The listing builds one solid part. Answer for the finished solid, in the listing's coordinates (mm). A direction names the side the tool comes from. Give positions to 0.01 mm unless a question says otherwise; leave off trailing zeros. Order: outer loops, then holes, each group sorted by start corner. A loop starts at its lowest first (then second) coordinate and runs counter-clockwise, first axis right, second up. Notation, with made-up numbers: (-31.5, 57) - (-15.5, 57) arc R34 ccw to (-15.5, 94) - close; hole circle Ø11 at (28, -0.5). An arc over 180 degrees is marked (long way). Answer as CSV lines item,"result". Start each with the question number.
1. Flat-ended cylindrical pins translate along their axes: pin 1 (0.5 mm diameter, centred on x = -3.5, y = -2, fed in from +Z); pin 2 (1.5 mm diameter, centred on x = -13, y = -2.5, fed in from -Z); pin 3 (2 mm diameter, centred on x = 32.5, y = -2, fed in from -Z); pin 4 (8 mm diameter, centred on x = -16, z = -41.5, fed in from -Y). Find the tip coordinate at first contact, or state that the pin passes through.
2. Which of the six approach directions +Z, -Z, +X, -X, +Y, -Y give full straight-line access (tool end or side, diameter ignored) to faces 1 (the cylindrical face through (-31.83, -3.05, 35.2)), 2 (the cylindrical face through (38.398, -0.673, -21.926)), 3 (the flat face through (0, -2, 46.1)), 4 (the cylindrical face through (31.83, -3.05, -35.2)), 5 (the flat face through (37.994, -0.159, -21.693))?
3. Section B-B on y = 1 is taken. Give the vertices of the cut face in (x, z) (3 decimals).
4. Determine the mould class of faces 6 (the flat face through (-39, -3.5, -23)), 7 (the flat face through (-38.347, -1.743, -22.382)), 8 (the conical face through (-22.56, 0.57, -38.24)) for opening direction Y: +Y half, -Y half, draft (parallel to the pull), parting line (faces both ways), or undercut.
5. Section A-A on x = 0 is taken. Give the vertices of the cut face in (y, z).
6. Section C-C on z = 0 is taken. Give the vertices of the cut face in (x, y).
7. Consider line 1 along Z through (x, y) = (7.5, -1.5); line 2 along X through (y, z) = (0.9, 0); line 3 along X through (y, z) = (0.7, 0). Determine where each line is inside the solid, lowest interval first. Write a range as [from, to].
from build123d import *

# Parameters (mm, degrees)
BOSS_EXTRUDE2_START       = -3.5
SKETCH1_W                 = 30
SKETCH1_H                 = 2.35
BOSS_EXTRUDE2_DEPTH       = 4.5
SKETCH3_R                 = 52.5
SKETCH3_R_2               = 42
SKETCH3_R_3               = 1.5
BOSS_EXTRUDE3_DEPTH       = 2
CHAMFER1_SIZE             = 3
CHAMFER1_SIZE_2           = 0.803847577
FILLET1_R                 = 1.5
F_1_0MM_START             = -15
F_1_0MM_DOWEL_SLOT1_DEPTH = 30
CIRPATTERN1_COUNT         = 6
FILLET1_OF_CIRPATTERN1_R  = 1.5


# Read off the part's stored shape, not the designer's step: Ø1.0mm Dowel Slot1
with BuildPart() as part:
    # Sketch1 → Boss-Extrude2 (new body)
    with BuildSketch(Plane(origin=(0, 0, 0), x_dir=(1, 0, 0), z_dir=(0, 1, 0)).offset(BOSS_EXTRUDE2_START)):
        with Locations((0, -44.925)):
            Rectangle(SKETCH1_W, SKETCH1_H)
    boss_extrude2 = extrude(amount=BOSS_EXTRUDE2_DEPTH)

    # Sketch3 → Boss-Extrude3 (add)
    with BuildSketch(Plane(origin=(0, 0, 0), x_dir=(1, 0, 0), z_dir=(0, 1, 0))):
        with Locations(Location((0, 0, 0), (0, 0, 270))):
            Circle(SKETCH3_R)
        with Locations(Location((0, 0, 0), (0, 0, 270))):
            Circle(SKETCH3_R_2, mode=Mode.SUBTRACT)
        with Locations(Location((-23.135, 40.070995433, 0), (0, 0, 270))):
            Circle(SKETCH3_R_3, mode=Mode.SUBTRACT)
        with Locations(Location((23.135, 40.070995433, 0), (0, 0, 270))):
            Circle(SKETCH3_R_3, mode=Mode.SUBTRACT)
        with Locations(Location((46.27, 0, 0), (0, 0, 270))):
            Circle(SKETCH3_R_3, mode=Mode.SUBTRACT)
        with Locations(Location((23.135, -40.070995433, 0), (0, 0, 270))):
            Circle(SKETCH3_R_3, mode=Mode.SUBTRACT)
        with Locations(Location((-23.135, -40.070995433, 0), (0, 0, 270))):
            Circle(SKETCH3_R_3, mode=Mode.SUBTRACT)
        with Locations(Location((-46.27, 0, 0), (0, 0, 270))):
            Circle(SKETCH3_R_3, mode=Mode.SUBTRACT)
    extrude(amount=BOSS_EXTRUDE3_DEPTH)

    # Chamfer1
    # the kernel refuses this chamfer: 3, 0.803847577 mm, written as the material it takes off along each edge
    with BuildSketch(Plane(origin=(23.135, 2, 40.070995433), x_dir=(0, 0, 1), z_dir=(-1, 0, 0))) as chamfer1_piece_1:
        Polygon((1.5, -CHAMFER1_SIZE), (1.5 + CHAMFER1_SIZE_2, 0), (1.5, 0), align=None)
    revolve(axis=Axis((23.135, 2, 40.070995433), (0, 1, 0)), mode=Mode.SUBTRACT)
    with BuildSketch(Plane(origin=(46.27, 2, 0), x_dir=(0, 0, 1), z_dir=(-1, 0, 0))) as chamfer1_piece_2:
        Polygon((1.5, -CHAMFER1_SIZE), (1.5 + CHAMFER1_SIZE_2, 0), (1.5, 0), align=None)
    revolve(axis=Axis((46.27, 2, 0), (0, 1, 0)), mode=Mode.SUBTRACT)
    with BuildSketch(Plane(origin=(23.135, 2, -40.070995433), x_dir=(0, 0, 1), z_dir=(-1, 0, 0))) as chamfer1_piece_3:
        Polygon((1.5, -CHAMFER1_SIZE), (1.5 + CHAMFER1_SIZE_2, 0), (1.5, 0), align=None)
    revolve(axis=Axis((23.135, 2, -40.070995433), (0, 1, 0)), mode=Mode.SUBTRACT)
    with BuildSketch(Plane(origin=(-23.135, 2, -40.070995433), x_dir=(0, 0, 1), z_dir=(-1, 0, 0))) as chamfer1_piece_4:
        Polygon((1.5, -CHAMFER1_SIZE), (1.5 + CHAMFER1_SIZE_2, 0), (1.5, 0), align=None)
    revolve(axis=Axis((-23.135, 2, -40.070995433), (0, 1, 0)), mode=Mode.SUBTRACT)
    with BuildSketch(Plane(origin=(-46.27, 2, 0), x_dir=(0, 0, 1), z_dir=(-1, 0, 0))) as chamfer1_piece_5:
        Polygon((1.5, -CHAMFER1_SIZE), (1.5 + CHAMFER1_SIZE_2, 0), (1.5, 0), align=None)
    revolve(axis=Axis((-46.27, 2, 0), (0, 1, 0)), mode=Mode.SUBTRACT)
    with BuildSketch(Plane(origin=(-23.135, 2, 40.070995433), x_dir=(0, 0, 1), z_dir=(-1, 0, 0))) as chamfer1_piece_6:
        Polygon((1.5, -CHAMFER1_SIZE), (1.5 + CHAMFER1_SIZE_2, 0), (1.5, 0), align=None)
    revolve(axis=Axis((-23.135, 2, 40.070995433), (0, 1, 0)), mode=Mode.SUBTRACT)

    # Fillet1
    fillet1_edges = [part.edges().sort_by_distance(p)[0] for p in [
        (-15, -3.5, 44.925),
        (15, -3.5, 44.925),
    ]]
    fillet(fillet1_edges, radius=FILLET1_R)

    # Ø1.0mm Dowel Slot1 outline → Ø1.0mm Dowel Slot1 (cut)
    with BuildSketch(Plane.YZ.offset(F_1_0MM_START)):
        with BuildLine():
            ThreePointArc((-0.3132503, 43.75), (-0.679912287, 44.221583836), (-1.25, 44.4))
            Line((-1.25, 44.4), (-2.25, 44.4))
            ThreePointArc((-2.25, 44.4), (-2.820087713, 44.221583836), (-3.1867497, 43.75))
            Line((-3.1867497, 43.75), (-0.3132503, 43.75))
        make_face()
    f_1_0mm_dowel_slot1 = extrude(amount=F_1_0MM_DOWEL_SLOT1_DEPTH, mode=Mode.SUBTRACT)

    # CirPattern1: Boss-Extrude2, Ø1.0mm Dowel Slot1 ×6 about axis
    cirpattern1_axis = Axis((0, 0, 0), (0, 1, 0))
    add([boss_extrude2.rotate(cirpattern1_axis, i * 360 / CIRPATTERN1_COUNT) for i in range(1, CIRPATTERN1_COUNT)])
    add([f_1_0mm_dowel_slot1.rotate(cirpattern1_axis, i * 360 / CIRPATTERN1_COUNT) for i in range(1, CIRPATTERN1_COUNT)], mode=Mode.SUBTRACT)

    # Fillet1 of CirPattern1
    fillet1_of_cirpattern1_edges = [part.edges().sort_by_distance(p)[0] for p in [
        (31.406191265, -3.5, 35.452881057),
        (46.406191265, -3.5, 9.472118943),
        (46.406191265, -3.5, -9.472118943),
        (31.406191265, -3.5, -35.452881057),
        (15, -3.5, -44.925),
        (-15, -3.5, -44.925),
        (-31.406191265, -3.5, -35.452881057),
        (-46.406191265, -3.5, -9.472118943),
        (-46.406191265, -3.5, 9.472118943),
        (-31.406191265, -3.5, 35.452881057),
    ]]
    fillet(fillet1_of_cirpattern1_edges, radius=FILLET1_OF_CIRPATTERN1_R)


solid = part.part
Checks:
1,pin 1,"stops at z = 46.1"
1,pin 2,"stops at z = -46.1"
1,pin 3,"stops at z = -36.04"
1,pin 4,"stops at y = -3.5"
2,face 1,"+Z, -Y"
2,face 2,"none"
2,face 3,"+Z, +X, -X, -Y"
2,face 4,"-Z, -Y"
2,face 5,"-Y"
3,outline,"circle Ø105 at (0, 0); hole circle Ø4.072 at (-46.27, 0); hole circle Ø84 at (0, 0); hole circle Ø4.072 at (-23.135, -40.071); hole circle Ø4.072 at (-23.135, 40.071); hole circle Ø4.072 at (23.135, -40.071); hole circle Ø4.072 at (23.135, 40.071); hole circle Ø4.072 at (46.27, 0)"
4,face 6,"-Y half"
4,face 7,"undercut"
4,face 8,"+Y half"
5,outline,"(-3.5, -46.1) - (0, -46.1) - (0, -52.5) - (2, -52.5) - (2, -42) - (0, -42) - (0, -43.75) - (-0.31, -43.75) arc R1 cw to (-1.25, -44.4) - (-2.25, -44.4) arc R1 cw to (-3.19, -43.75) - (-3.5, -43.75) - close; (-3.5, 43.75) - (-3.19, 43.75) arc R1 cw to (-2.25, 44.4) - (-1.25, 44.4) arc R1 cw to (-0.31, 43.75) - (0, 43.75) - (0, 42) - (2, 42) - (2, 52.5) - (0, 52.5) - (0, 46.1) - (-3.5, 46.1) - close"
6,outline,"(-52.5, 0) - (-48.04, 0) - (-48.57, 2) - (-52.5, 2) - close; (-44.5, 0) - (-42, 0) - (-42, 2) - (-43.97, 2) - close; (42, 0) - (44.5, 0) - (43.97, 2) - (42, 2) - close; (48.04, 0) - (52.5, 0) - (52.5, 2) - (48.57, 2) - close"
7,line 1,"z = [-46.1, -44.4], [44.4, 46.1]"
7,line 2,"x = [-52.5, -48.28], [-44.26, -42], [42, 44.26], [48.28, 52.5]"
7,line 3,"x = [-52.5, -48.23], [-44.31, -42], [42, 44.31], [48.23, 52.5]"
